Autodesk Inventor part; units mm, degrees
ref_plane "YZ Plane" through (0, 0, 0) normal (1, 0, 0) x (0, 1, 0)
ref_plane "XZ Plane" through (0, 0, 0) normal (0, 1, 0) x (-1, 0, 0)
ref_plane "XY Plane" through (0, 0, 0) normal (0, 0, 1) x (1, 0, 0)
sketch "Sketch1" plane through (0, 0, 0) normal (0, 0, 1) x (1, 0, 0)
  line L0 (44.45, -76.9897) -> (-44.45, -76.9897)
  line L1 (-44.45, -76.9897) -> (-88.9, 0)
  line L2 (-88.9, 0) -> (-44.45, 76.9897)
  line L3 (-44.45, 76.9897) -> (44.45, 76.9897)
  line L4 (44.45, 76.9897) -> (88.9, 0)
  line L5 (88.9, 0) -> (44.45, -76.9897)
  circle A0 centre (0, 0) radius 25.4
  line L6 (0, 107.7855) -> (0, -107.7855)
  line L7 (-124.46, 0) -> (124.46, 0)
  point P0 (0, 0)
  point P1 (0, 0)
  dimension "d1" = 88.9
  dimension "d4" = 50.8
  dimension "d7" = 88.9
  dimension "d8" = 88.9
  dimension "d9" = 88.9
  dimension "d10" = 120
  dimension "d11" = 120
  dimension "d12" = 120
  dimension "d13" = 120
  dimension "d14" = 120
  dimension "d15" = 44.45
extrude "Extrusion1" add sketch "Sketch1" along normal blind 28.448
sketch "Sketch2" plane through (0, 0, 0) normal (0, 0, -1) x (-1, 0, 0)
  line L0 (-44.45, -76.9897) -> (44.45, -76.9897)
  line L1 (44.45, -76.9897) -> (88.9, 0)
  line L2 (88.9, 0) -> (44.45, 76.9897)
  line L3 (44.45, 76.9897) -> (-44.45, 76.9897)
  line L4 (-44.45, 76.9897) -> (-88.9, 0)
  line L5 (-88.9, 0) -> (-44.45, -76.9897)
  circle A0 centre (0, 0) radius 25.4
  point P0 (0, 0)
  point P1 (0, 0)
extrude "Extrusion2" cut sketch "Sketch1" along normal blind 44.45 contours L6 L7 A0 | A0 L7 L6 | L7 L6 A0 | A0 L6 L7
sketch "Sketch3" plane through (0, 0, 28.448) normal (0, 0, 1) x (1, 0, 0)
  line L0 (0, 107.7855) -> (0, -107.7855)
  line L1 (-124.46, 0) -> (124.46, 0)
  line L2 (28.194, 47.244) -> (28.194, -47.244) construction
  line L3 (28.194, -47.244) -> (-28.194, -47.244) construction
  line L4 (-28.194, -47.244) -> (-28.194, 47.244) construction
  line L5 (-28.194, 47.244) -> (28.194, 47.244) construction
  line L6 (28.194, 47.244) -> (-28.194, -47.244) construction
  line L7 (28.194, -47.244) -> (-28.194, 47.244) construction
  point P0 (0, 0)
  point P1 (0, 47.244)
  point P2 (0, -47.244)
  dimension "d16" = 56.388
  dimension "d17" = 94.488
  dimension "d18" = 0
hole "Hole1" at (-28.194, 47.244, 28.448) at (28.194, 47.244, 28.448) at (28.194, -47.244, 28.448) at (-28.194, -47.244, 28.448) at (0, 47.244, 28.448) at (0, -47.244, 28.448) direction (0, 0, -1) diameter 3.302 end through all
properties part number "JF-AT-TM0009" material "Acrylic, Clear"
Design review of the part built by this model. Coordinates are the model's own, in mm. Coordinates: 2 decimals unless noted, no trailing zeros. Write each loop counter-clockwise with the first axis right and the second up, starting at its lowest first coordinate (ties: lowest second). Pieces come first, ordered by that corner, then holes. Notation, with made-up numbers: (-25, 51) -> (-1, 51) arc R13 ccw to (-1, 58) -> close; hole circle Ø1 at (71, -26.5). An arc over 180 degrees is marked (long way). Write each question's results on one line, items separated by ' | '. Start each with the question number.
(1) Take a section at B-B on z = 4. Write out the cut boundary in (x, y) (3 decimals), and give its area (3 significant figures).
(2) Take a section at C-C on y = -13.5. Write out the cut boundary in (x, z), and give its area (3 significant figures).
(3) Take a section at D-D on y = -57.5. Write out the cut boundary in (x, z).
(4) For line 1 along Y through (x, z) = (0, 18.25) (3 decimals); line 2 along X through (y, z) = (-8, 27.25); line 3 along Y through (x, z) = (5, 13), list the stretches that pass through material, from the lowest coordinate up. Write a range as from..to.
(5) The part is to be moulded in two halves that separate along Y. For faces 1 (the face through (-5.506, 24.796, 14.025)), 2 (the face through (19, 18, 0)), 3 (the face through (-66.364, -39.034, 14.025)), say which applies: pulls with the +Y half, pulls with the -Y half, needs draft (parallel to the pull), parting line crosses it, or undercut.
(6) Clearance check with flat-ended pins moving along their axes: P1, Ø3, axis at x = -65.5, z = 17, coming from the +Y side; P2, Ø8, axis at y = 57, z = 6, coming from the -X side; P3, Ø4, axis at x = -51.5, z = 23, coming from the -Y side. State where each tip first meets the part, or that it passes through.
(7) Take a section at A-A on x = 4.5. Write out the cut boundary in (y, z), and give its area (3 significant figures).
Results found:
1) outline: (-88.9, 0) -> (-44.45, -76.99) -> (44.45, -76.99) -> (88.9, 0) -> (44.45, 76.99) -> (-44.45, 76.99) -> close; hole circle Ø3.302 at (-28.194, -47.244); hole circle Ø3.302 at (-28.194, 47.244); hole circle Ø50.8 at (0, 0); hole circle Ø3.302 at (0, -47.244); hole circle Ø3.302 at (0, 47.244); hole circle Ø3.302 at (28.194, -47.244); hole circle Ø3.302 at (28.194, 47.244) | area: 18,500 mm2
2) outline: (-81.11, 0) -> (-21.52, 0) -> (-21.52, 28.45) -> (-81.11, 28.45) -> close; (21.52, 0) -> (81.11, 0) -> (81.11, 28.45) -> (21.52, 28.45) -> close | area: 3,390 mm2
3) outline: (-55.7, 0) -> (55.7, 0) -> (55.7, 28.45) -> (-55.7, 28.45) -> close
4) line 1: y = -76.99..-48.895, -45.593..-25.4, 25.4..45.593, 48.895..76.99 | line 2: x = -84.28..-24.11, 24.11..84.28 | line 3: y = -76.99..-24.9, 24.9..76.99
5) face 1: undercut | face 2: needs draft | face 3: pulls with the -Y half
6) P1: stops at y = 43.13 | P2: stops at x = -58.3 | P3: stops at y = -68.24
7) outline: (-76.99, 0) -> (-25, 0) -> (-25, 28.45) -> (-76.99, 28.45) -> close; (25, 0) -> (76.99, 0) -> (76.99, 28.45) -> (25, 28.45) -> close | area: 2,960 mm2
